from build123d import *

# Parameters (mm, degrees)
BOSS_EXTRUDE1_DEPTH = 2
FILLET5_R           = 0.3
FILLET7_R           = 0.3
FILLET8_R           = 0.3
FILLET9_R           = 0.3
FILLET10_R          = 0.3
FILLET11_R          = 0.3


with BuildPart() as part:
    # Sketch1 → Boss-Extrude1 (new body)
    with BuildSketch(Plane.XY):
        Polygon((-24.5, -2.5), (-24.5, -4.5), (25.5, -4.5), (25.5, -2.5), (27.5, -2.5), (27.5, 2.5), (25.5, 2.5), (25.5, 4.5), (-24.5, 4.5), (-24.5, 2.5), (-27.5, 2.5), (-27.5, -2.5), align=None)
    extrude(amount=BOSS_EXTRUDE1_DEPTH)

    # Fillet5
    fillet5_edges = [part.edges().sort_by_distance(p)[0] for p in [
        (-27.5, -2.5, 1),
    ]]
    fillet(fillet5_edges, radius=FILLET5_R)

    # Fillet7
    fillet7_edges = [part.edges().sort_by_distance(p)[0] for p in [
        (-24.5, -4.5, 1),
    ]]
    fillet(fillet7_edges, radius=FILLET7_R)

    # Fillet8
    fillet8_edges = [part.edges().sort_by_distance(p)[0] for p in [
        (-24.5, 4.5, 1),
    ]]
    fillet(fillet8_edges, radius=FILLET8_R)

    # Fillet9
    fillet9_edges = [part.edges().sort_by_distance(p)[0] for p in [
        (25.5, -4.5, 1),
    ]]
    fillet(fillet9_edges, radius=FILLET9_R)

    # Fillet10
    fillet10_edges = [part.edges().sort_by_distance(p)[0] for p in [
        (25.5, 4.5, 1),
        (27.5, 2.5, 1),
        (27.5, -2.5, 1),
    ]]
    fillet(fillet10_edges, radius=FILLET10_R)

    # Fillet11
    fillet11_edges = [part.edges().sort_by_distance(p)[0] for p in [
        (-27.5, 2.5, 1),
    ]]
    fillet(fillet11_edges, radius=FILLET11_R)


solid = part.part
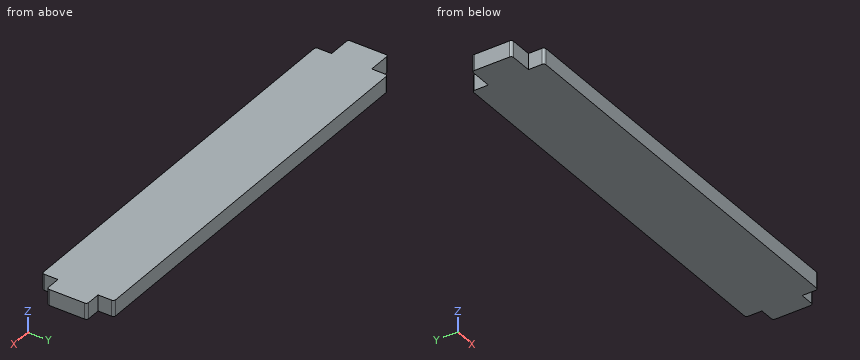
Verification items for the finished model (mm, model axes). Round coordinates to 2 decimals unless told otherwise and drop trailing zeros. Loops run counter-clockwise (first coordinate to the right, second up) from the corner with the lowest first, then second, coordinate; pieces in that order, holes last. Notation, with made-up numbers: (5.25, -18) - (61.25, -18) arc R25 ccw to (61.25, 17) - close; hole circle Ø2 at (79, 60.25). An arc over 180 degrees is marked (long way). Answer in a Markdown table with one row per item. Add a question column.
Q1. Section check B-B on y = 3.25. Enter the section's corners in (x, z), plus the area to 3 significant figures.
Q2. Material ranges on line 1 (X direction, y = -2.75, z = 1.05); line 2 (X direction, y = -2.25, z = 0.1), recorded low to high.
Q3. Section check A-A on z = 0.85. Enter the section's corners in (x, y), plus the area to 3 significant figures.
Q4. Gauge pin test, flat ends, axial feed: pin 1 (5 mm diameter, centred on x = 6.5, y = 1.5, fed in from -Z); pin 2 (0.8 mm diameter, centred on x = 27, z = 1, fed in from +Y); pin 3 (0.5 mm diameter, centred on x = 26, z = 1, fed in from -Y); pin 4 (1 mm diameter, centred on y = 3.5, z = 1, fed in from -X). Record the tip position at first contact, or that the pin passes through.
Found:
| question | item | result |
|---|---|---|
| 1 | outline | (-24.5, 0) - (25.5, 0) - (25.5, 2) - (-24.5, 2) - close |
| 1 | area | 100 mm² |
| 2 | line 1 | x = -24.5 to 25.5 |
| 2 | line 2 | x = -27.5 to 27.5 |
| 3 | outline | (-27.5, -2.2) arc R0.3 ccw to (-27.2, -2.5) - (-24.5, -2.5) - (-24.5, -4.2) arc R0.3 ccw to (-24.2, -4.5) - (25.2, -4.5) arc R0.3 ccw to (25.5, -4.2) - (25.5, -2.5) - (27.2, -2.5) arc R0.3 ccw to (27.5, -2.2) - (27.5, 2.2) arc R0.3 ccw to (27.2, 2.5) - (25.5, 2.5) - (25.5, 4.2) arc R0.3 ccw to (25.2, 4.5) - (-24.2, 4.5) arc R0.3 ccw to (-24.5, 4.2) - (-24.5, 2.5) - (-27.2, 2.5) arc R0.3 ccw to (-27.5, 2.2) - close |
| 3 | area | 475 mm² |
| 4 | pin 1 | stops at z = 0 |
| 4 | pin 2 | stops at y = 2.5 |
| 4 | pin 3 | stops at y = -2.5 |
| 4 | pin 4 | stops at x = -24.5 |
